Could you check a few things on this model? Use its own coordinates, in mm. Face numbers are marked on the shaded views. A direction names the side the tool comes from. Coordinates: 2 decimals unless noted, no trailing zeros. Order: outer loops, then holes, each group sorted by start corner. A loop starts at its lowest first (then second) coordinate and runs counter-clockwise, first axis right, second up. Notation, with made-up numbers: (-19, 25.25) -> (4, 25.25) arc R18 ccw to (4, 41.25) -> close; hole circle Ø9 at (-31.75, 26.25). An arc over 180 degrees is marked (long way). Put each result on its own line as item: value. Start each with the question number.
Q1. Please list where these lines run through material, in increasing order: line 1 along X through (y, z) = (7, 5); line 2 along Y through (x, z) = (-15, 21); line 3 along Z through (x, y) = (21, -17.5).
Q2. If we section it at A-A (z = -18): Please give me the cut outline in (x, y), and give its area (3 significant figures).
Q3. If we section it at C-C (x = 6): Please give me the cut outline in (y, z).
Q4. We'd pull the mould along X, two halves only. Please class the marked faces 3, 4, 5 and 6: +X half, -X half, draft (parallel to the pull), parting line (faces both ways), or undercut.
Q5. If we section it at D-D (z = 10.5): Please give me the cut outline in (x, y), and give its area (3 significant figures).
Q6. If we section it at B-B (y = 6): Please give me the cut outline in (x, z).
Q7. For the marked faces 1 and 2, which set-ups out of +Z, -Z, +X, -X, +Y, -Y let a thin tool reach every point of the face, with its end or its side?
Q8. Will these pins go through, and if not, where does the flat tip stop? pin 1 (8 mm diameter, centred on x = -34, z = 22.5, fed in from +Y); pin 2 (0.8 mm diameter, centred on y = -26, z = -14.5, fed in from -X).
from build123d import *

# Parameters (mm, degrees)
F0_W          = 41.1777616951
F0_H          = 58.2677274942
F1_DEPTH      = 25
F1_DEPTH_BACK = 25
F2_DEPTH      = 26.5
F2_DEPTH_BACK = 26.75
F3_R          = 21
F4_R          = 21


with BuildPart() as f1:
    # F0 (on Front) → F1 (new body, two sides)
    with BuildSketch(Plane.XZ) as f1_sk:
        with Locations((-26.726005576, 0)):
            Rectangle(F0_W, F0_H)
    extrude(amount=F1_DEPTH)
    extrude(f1_sk.sketch, amount=-F1_DEPTH_BACK)

    # F0 (on Front) → F2 (join, two sides)
    with BuildSketch(Plane.XZ) as f2_sk:
        with BuildLine():
            Line((47.3148864236, 29.1338637471), (-6.1371247284, 29.1338637471))
            Line((-6.1371247284, 29.1338637471), (-6.1371247284, -29.1338637471))
            Line((-6.1371247284, -29.1338637471), (3.736696206, -29.1338637471))
            Line((3.736696206, -29.1338637471), (3.736696206, 5.2775406944))
            ThreePointArc((3.736696206, 5.2775406944), (20.2848818153, 20.1810889299), (36.8330674246, 5.2775406944))
            Line((36.8330674246, 5.2775406944), (36.8330674246, -29.1338637471))
            Line((36.8330674246, -29.1338637471), (47.3148864236, -29.1338637471))
            Line((47.3148864236, -29.1338637471), (47.3148864236, 29.1338637471))
        make_face()
    extrude(amount=F2_DEPTH)
    extrude(f2_sk.sketch, amount=-F2_DEPTH_BACK)

    # F3
    f3_edges = [f1.edges().sort_by_distance(p)[0] for p in [
        (-6.137125, -25.75, 29.133864),
    ]]
    fillet(f3_edges, radius=F3_R)

    # F4
    f4_edges = [f1.edges().sort_by_distance(p)[0] for p in [
        (-6.137125, 25.875, 29.133864),
    ]]
    fillet(f4_edges, radius=F4_R)


solid = f1.part
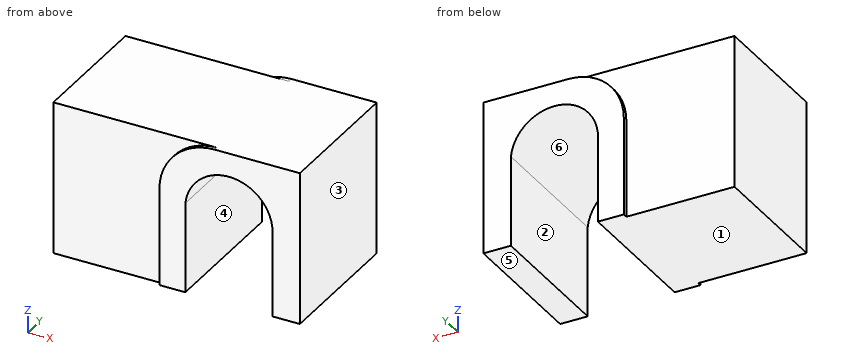
The answers:
1. line 1: -47.31 to 3.74, 36.83 to 47.31
1. line 2: -25 to 25
1. line 3: 20.17 to 29.13
2. outline: (-47.31, -25) -> (-6.14, -25) -> (-6.14, -26.5) -> (3.74, -26.5) -> (3.74, 26.75) -> (-6.14, 26.75) -> (-6.14, 25) -> (-47.31, 25) -> close; (36.83, -26.5) -> (47.31, -26.5) -> (47.31, 26.75) -> (36.83, 26.75) -> close
2. area: 3,140 mm^2
3. outline: (-26.5, 12.07) -> (26.75, 12.07) -> (26.75, 27.17) -> (25, 27.17) -> (25, 29.13) -> (-25, 29.13) -> (-25, 27.17) -> (-26.5, 27.17) -> close
4. face 3: +X half
4. face 4: undercut
4. face 5: draft
4. face 6: undercut
5. outline: (-47.31, -25) -> (-6, -25) -> (-6, -26.5) -> (5.17, -26.5) -> (5.17, 26.75) -> (-6, 26.75) -> (-6, 25) -> (-47.31, 25) -> close; (35.4, -26.5) -> (47.31, -26.5) -> (47.31, 26.75) -> (35.4, 26.75) -> close
5. area: 3,300 mm^2
6. outline: (-47.31, -29.13) -> (3.74, -29.13) -> (3.74, 5.28) arc R16.64 cw to (36.83, 5.28) -> (36.83, -29.13) -> (47.31, -29.13) -> (47.31, 29.13) -> (-47.31, 29.13) -> close
7. face 1: -Z, +X, -X, +Y, -Y
7. face 2: -Z, +Y, -Y
8. pin 1: y = 25
8. pin 2: x = -6.14
